Input: dimensioned drawing with shaded views. Units: mm. Origin: part minimum x, y, z. Give positions to 0.01 mm unless a question says otherwise; leave off trailing zeros. Order: outer loops, then holes, each group sorted by start corner. A loop starts at its lowest first (then second) coordinate and runs counter-clockwise, first axis right, second up. Notation, with made-up numbers: (5.25, 80) -> (33.25, 80) arc R23 ccw to (33.25, 107) -> close; hole circle Ø6 at (-29.75, 39.25). An arc over 180 degrees is marked (long way). Use CSV: the item, a comma, the result in double quotes.
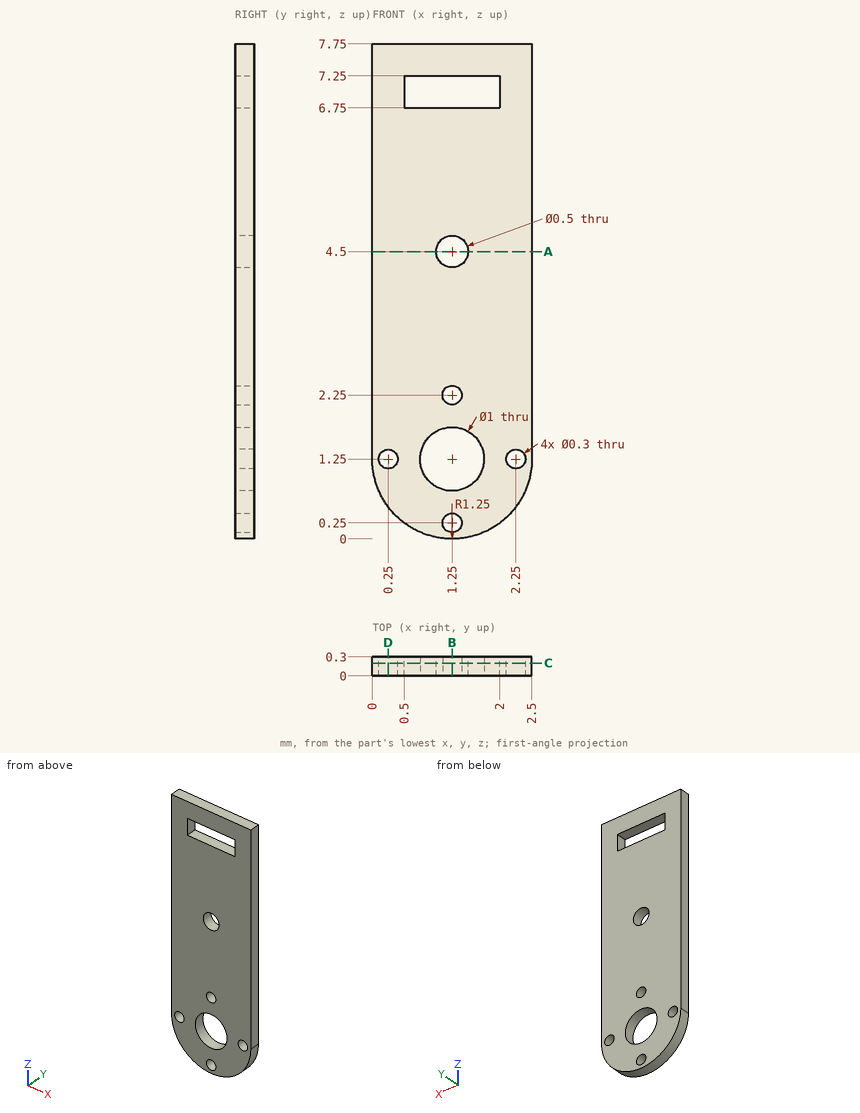
1. Ray query, line 1 along Z through (x, y) = (0.9, 0.25); line 2 along X through (y, z) = (0.25, 0.25); line 3 along X through (y, z) = (0.1, 2.25). Return the intervals inside material, ascending.
Answer below:
line 1,"z = 0.05 to 0.89, 1.61 to 6.75, 7.25 to 7.75"
line 2,"x = 0.5 to 1.1, 1.4 to 2"
line 3,"x = 0 to 1.1, 1.4 to 2.5"
2. Section query B-B on x = 1.25. Return loops of the section in (y, z), plus the area to 4 significant figures.
Answer below:
outline,"(0, 0) -> (0.3, 0) -> (0.3, 0.1) -> (0, 0.1) -> close; (0, 0.4) -> (0.3, 0.4) -> (0.3, 0.75) -> (0, 0.75) -> close; (0, 1.75) -> (0.3, 1.75) -> (0.3, 2.1) -> (0, 2.1) -> close; (0, 2.4) -> (0.3, 2.4) -> (0.3, 4.25) -> (0, 4.25) -> close; (0, 4.75) -> (0.3, 4.75) -> (0.3, 6.75) -> (0, 6.75) -> close; (0, 7.25) -> (0.3, 7.25) -> (0.3, 7.75) -> (0, 7.75) -> close"
area,"1.545 mm²"
3. Section query C-C on y = 0.2. Return loops of the section in (x, z).
Answer below:
outline,"(0, 1.25) arc R1.25 ccw to (2.5, 1.25) -> (2.5, 7.75) -> (0, 7.75) -> close; hole circle Ø0.3 at (0.25, 1.25); hole (0.5, 6.75) -> (2, 6.75) -> (2, 7.25) -> (0.5, 7.25) -> close; hole circle Ø1 at (1.25, 1.25); hole circle Ø0.5 at (1.25, 4.5); hole circle Ø0.3 at (1.25, 0.25); hole circle Ø0.3 at (1.25, 2.25); hole circle Ø0.3 at (2.25, 1.25)"
4. Pin query (flat end, axial travel): P1, Ø1, axis at x = 0.5, z = 3, coming from the -Y side. Return the tip coordinate at first contact, or that it passes through.
Answer below:
P1,"stops at y = 0"
5. Section query A-A on z = 4.5. Return loops of the section in (x, y).
Answer below:
outline,"(0, 0) -> (1, 0) -> (1, 0.3) -> (0, 0.3) -> close; (1.5, 0) -> (2.5, 0) -> (2.5, 0.3) -> (1.5, 0.3) -> close"
6. Section query D-D on x = 0.25. Return loops of the section in (y, z), plus the area to 4 significant figures.
Answer below:
outline,"(0, 0.5) -> (0.3, 0.5) -> (0.3, 1.1) -> (0, 1.1) -> close; (0, 1.4) -> (0.3, 1.4) -> (0.3, 7.75) -> (0, 7.75) -> close"
area,"2.085 mm²"
